Could you check a few things on this model? Use its own coordinates, in mm. A direction names the side the tool comes from. Coordinates: 2 decimals unless noted, no trailing zeros. Loops run counter-clockwise (first coordinate to the right, second up) from the corner with the lowest first, then second, coordinate; pieces in that order, holes last.
1) Imagine slicing it at D-D on y = -33.5. Please give me the cut outline in (x, z).
2) For faces 1 (the face through (6.4, -31.8, 6.4)), 2 (the face through (6, -15, 12.7)), which set-ups out of +Z, -Z, +X, -X, +Y, -Y let a thin tool reach every point of the face, with its end or its side?
3) If I drill on line 1 along X through (y, z) = (-17.5, 26); line 2 along Z through (x, y) = (11.25, -9); line 3 along Y through (x, z) = (22.5, 22.5), over which ranges is the centre line in solid material (lowest first)?
4) Will these pins go through, and if not, where does the flat tip stop? P1, Ø10, axis at x = 4.5, y = -13.5, coming from the +Z side; P2, Ø8, axis at x = 21, z = 19, coming from the -Y side; P3, Ø2, axis at x = 20, y = -25, coming from the +Z side.
5) Imagine slicing it at C-C on z = 7. Please give me the cut outline in (x, y), plus the area to 3 significant figures.
6) Imagine slicing it at A-A on y = -28. Please give me the cut outline in (x, z), plus the area to 3 significant figures.
7) Imagine slicing it at B-B on x = 14.75. Please give me the cut outline in (y, z), plus the area to 3 significant figures.
```python
from build123d import *

# Parameters (mm, degrees)
F0_W     = 25.4
F0_H     = 31.75
F1_DEPTH = 38.1
F2_W     = 12.7
F2_H     = 19.05
F3_DEPTH = 38.1
F5_DEPTH = 25.4
F7_DEPTH = 25.4


with BuildPart() as f1:
    # F0 (on Front) → F1 (new body)
    with BuildSketch(Plane.XZ):
        with Locations((12.7, 15.875)):
            Rectangle(F0_W, F0_H)
    extrude(amount=F1_DEPTH)

    # F2 (on face) → F3 (cut)
    with BuildSketch(Plane.XZ.offset(38.1)):
        with Locations((6.35, 22.225)):
            Rectangle(F2_W, F2_H)
    extrude(amount=-F3_DEPTH, mode=Mode.SUBTRACT)

    # F4 (on face) → F5 (cut)
    with BuildSketch(Plane(origin=(12.7, 0, 0), x_dir=(0, -1, 0), z_dir=(-1, 0, 0))):
        Polygon((38.1, 12.7), (38.1, 31.75), (19.05, 31.75), align=None)
    extrude(amount=-F5_DEPTH, mode=Mode.SUBTRACT)

    # F6 (on face) → F7 (cut)
    with BuildSketch(Plane.XY.offset(12.7)):
        Polygon((0, -25.4), (0, -38.1), (12.7, -38.1), align=None)
    extrude(amount=-F7_DEPTH, mode=Mode.SUBTRACT)


solid = f1.part
```
Filled in:
1. outline: (8.1, 0) - (25.4, 0) - (25.4, 17.3) - (12.7, 17.3) - (12.7, 12.7) - (8.1, 12.7) - close
2. face 1: +Z, -Z, -X, -Y
2. face 2: +Z, -X, +Y, -Y
3. line 1: x = 12.7 to 25.4
3. line 2: z = 0 to 12.7
3. line 3: y = -28.3 to 0
4. P1: stops at z = 12.7
4. P2: stops at y = -35.8
4. P3: stops at z = 26.8
5. outline: (0, -25.4) - (12.7, -38.1) - (25.4, -38.1) - (25.4, 0) - (0, 0) - close
5. area: 887 mm2
6. outline: (2.6, 0) - (25.4, 0) - (25.4, 22.8) - (12.7, 22.8) - (12.7, 12.7) - (2.6, 12.7) - close
6. area: 418 mm2
7. outline: (-38.1, 0) - (0, 0) - (0, 31.75) - (-19.05, 31.75) - (-38.1, 12.7) - close
7. area: 1,030 mm2
